Model file for the job. Use its own axes, mm. A direction names the side the tool comes from. Round coordinates to 2 decimals unless told otherwise and drop trailing zeros. Order: outer loops, then holes, each group sorted by start corner. A loop starts at its lowest first (then second) coordinate and runs counter-clockwise, first axis right, second up. Notation, with made-up numbers: (-27, -10) -> (-20, -10) arc R22 ccw to (-20, 27) -> close; hole circle Ø3 at (-19, 7). An arc over 180 degrees is marked (long way). Use CSV: the item, a comma, the result in double quotes.
```python
from build123d import *

# Parameters (mm, degrees)
BOSS_EXTRUDE1_DEPTH = 24
SKETCH2_R           = 2.05
SKETCH2_R_2         = 4
CUT_EXTRUDE1_DEPTH  = 43.755116653
SKETCH3_R           = 4
SKETCH3_R_2         = 2
CUT_EXTRUDE2_DEPTH  = 43.755116653
FILLET1_R           = 2


with BuildPart() as part:
    # Sketch1 → Boss-Extrude1 (new body)
    with BuildSketch(Plane.XY):
        Polygon((0, 0), (0, 26), (2, 26), (2, 2), (26, 2), (26, 0), align=None)
    extrude(amount=BOSS_EXTRUDE1_DEPTH)

    # Sketch2 → Cut-Extrude1 (cut, through all)
    with BuildSketch(Plane(origin=(2, 0, 0), x_dir=(0, 0, -1), z_dir=(1, 0, 0))):
        with Locations(Location((-12, 22, 0), (0, 0, 90))):
            Circle(SKETCH2_R)
        with Locations(Location((-12, 14, 0), (0, 0, 90))):
            Circle(SKETCH2_R_2)
        with Locations(Location((-6.343145751, 19.656854249, 0), (0, 0, 90))):
            Circle(SKETCH2_R)
        with Locations(Location((-4, 14, 0), (0, 0, 90))):
            Circle(SKETCH2_R)
        with Locations(Location((-6.343145751, 8.343145751, 0), (0, 0, 90))):
            Circle(SKETCH2_R)
        with Locations(Location((-12, 6, 0), (0, 0, 90))):
            Circle(SKETCH2_R)
        with Locations(Location((-17.656854249, 8.343145751, 0), (0, 0, 90))):
            Circle(SKETCH2_R)
        with Locations(Location((-20, 14, 0), (0, 0, 90))):
            Circle(SKETCH2_R)
        with Locations(Location((-17.656854249, 19.656854249, 0), (0, 0, 90))):
            Circle(SKETCH2_R)
    extrude(amount=-CUT_EXTRUDE1_DEPTH, mode=Mode.SUBTRACT)

    # Sketch3 → Cut-Extrude2 (cut, through all)
    with BuildSketch(Plane(origin=(0, 2, 0), x_dir=(1, 0, 0), z_dir=(0, 1, 0))):
        with Locations(Location((14, -12, 0), (0, 0, 270))):
            Circle(SKETCH3_R)
        with Locations(Location((22, -12, 0), (0, 0, 270))):
            Circle(SKETCH3_R_2)
        with Locations(Location((19.656854249, -17.656854249, 0), (0, 0, 270))):
            Circle(SKETCH3_R_2)
        with Locations(Location((14, -20, 0), (0, 0, 270))):
            Circle(SKETCH3_R_2)
        with Locations(Location((8.343145751, -17.656854249, 0), (0, 0, 270))):
            Circle(SKETCH3_R_2)
        with Locations(Location((6, -12, 0), (0, 0, 270))):
            Circle(SKETCH3_R_2)
        with Locations(Location((8.343145751, -6.343145751, 0), (0, 0, 270))):
            Circle(SKETCH3_R_2)
        with Locations(Location((14, -4, 0), (0, 0, 270))):
            Circle(SKETCH3_R_2)
        with Locations(Location((19.656854249, -6.343145751, 0), (0, 0, 270))):
            Circle(SKETCH3_R_2)
    extrude(amount=-CUT_EXTRUDE2_DEPTH, mode=Mode.SUBTRACT)

    # Fillet1
    fillet1_edges = [part.edges().sort_by_distance(p)[0] for p in [
        (1, 26, 24),
        (1, 26, 0),
        (26, 1, 24),
        (26, 1, 0),
    ]]
    fillet(fillet1_edges, radius=FILLET1_R)


solid = part.part
```
Q1. Pin check, flat tips, straight feed: pin 1 (12 mm diameter, centred on y = 9, z = 17.5, fed in from +X); pin 2 (2.5 mm diameter, centred on y = 6, z = 12, fed in from -X); pin 3 (4.5 mm diameter, centred on x = 8.34, z = 17.66, fed in from +Y). Stop position of each tip, or through.
From the geometry:
pin 1,"stops at x = 2"
pin 2,"passes through"
pin 3,"stops at y = 2"
Q2. Cut at D-D (x = 9). Give the cut face in (y, z).
From the geometry:
outline,"(0, 0) -> (2, 0) -> (2, 4.45) -> (0, 4.45) -> close; (0, 8.23) -> (2, 8.23) -> (2, 15.77) -> (0, 15.77) -> close; (0, 19.55) -> (2, 19.55) -> (2, 24) -> (0, 24) -> close"
Q3. Cut at B-B (x = 14). Give the cut face in (y, z), plus the area to 3 significant figures.
From the geometry:
outline,"(0, 0) -> (2, 0) -> (2, 2) -> (0, 2) -> close; (0, 6) -> (2, 6) -> (2, 8) -> (0, 8) -> close; (0, 16) -> (2, 16) -> (2, 18) -> (0, 18) -> close; (0, 22) -> (2, 22) -> (2, 24) -> (0, 24) -> close"
area,"16.0 mm²"
Q4. Cut at A-A (y = 14). Give the cut face in (x, z), plus the area to 3 significant figures.
From the geometry:
outline,"(0, 0) -> (2, 0) -> (2, 1.95) -> (0, 1.95) -> close; (0, 6.05) -> (2, 6.05) -> (2, 8) -> (0, 8) -> close; (0, 16) -> (2, 16) -> (2, 17.95) -> (0, 17.95) -> close; (0, 22.05) -> (2, 22.05) -> (2, 24) -> (0, 24) -> close"
area,"15.6 mm²"
Q5. Cut at C-C (z = 17). Give the cut face in (x, y).
From the geometry:
outline,"(0, 0) -> (6.45, 0) -> (6.45, 2) -> (2, 2) -> (2, 6.4) -> (0, 6.4) -> close; (0, 10.29) -> (2, 10.29) -> (2, 17.71) -> (0, 17.71) -> close; (0, 21.6) -> (2, 21.6) -> (2, 26) -> (0, 26) -> close; (10.23, 0) -> (17.77, 0) -> (17.77, 2) -> (10.23, 2) -> close; (21.55, 0) -> (26, 0) -> (26, 2) -> (21.55, 2) -> close"
Q6. Mould opens along Y. For faces 1 (the cylindrical face through (1.01, 25.4, 23.43)), 2 (the cylindrical face through (1.014, 9.445, 19.385)), 3 (the cylindrical face through (6, 1, 10)) say: +Y half, -Y half, draft (parallel to the pull), parting line (faces both ways), or undercut.
From the geometry:
face 1,"+Y half"
face 2,"undercut"
face 3,"draft"
Q7. Which spindle directions (+Z, -Z, +X, -X, +Y, -Y) get a long thin tool onto all of the face, cutting with end or side? Do faces 4 (the cylindrical face through (17.883, 1.014, 18.58)), 5 (the flat face through (2, 17, 9)). Say none if no direction does.
From the geometry:
face 4,"+Y, -Y"
face 5,"+Z, -Z, +X, +Y"
Q8. Probe line 1 along X through (y, z) = (1.55, 12); line 2 along Z through (x, y) = (1.05, 22); line 3 along Y through (x, z) = (1.75, 19.25). List the from-to ranges inside material, lowest first.
From the geometry:
line 1,"x = 0 to 4, 8 to 10, 18 to 20, 24 to 26"
line 2,"z = 0 to 9.95, 14.05 to 24"
line 3,"y = 0 to 7.05, 9.63 to 12.09, 15.91 to 18.37, 20.95 to 26"
